Here's how the part is built. I have some questions about the finished solid (model axes, mm). A direction names the side the tool comes from. Coordinates: 2 decimals unless noted, no trailing zeros. Write each loop counter-clockwise with the first axis right and the second up, starting at its lowest first coordinate (ties: lowest second). Pieces come first, ordered by that corner, then holes. Notation, with made-up numbers: (0, -16.75) -> (26, -16.75) arc R16 ccw to (26, 1.25) -> close; hole circle Ø3 at (24, 88). An arc over 180 degrees is marked (long way). Use a Markdown table: item, result. Add a question column.
```python
from build123d import *

# Parameters (mm, degrees)
F0_R      = 12
F1_DEPTH  = 100
F2_R      = 10
F3_DEPTH  = 100
F4_R      = 32
F4_R_2    = 12
F5_DEPTH  = 5
F6_R      = 32
F6_R_2    = 12
F7_DEPTH  = 5
F8_R      = 5
F9_DEPTH  = 100
F14_R     = 5
F15_DEPTH = 50
F16_R     = 10
F17_DEPTH = 70


with BuildPart() as f1:
    # F0 (on Top) → F1 (new body)
    with BuildSketch(Plane.XY):
        Circle(F0_R)
    extrude(amount=F1_DEPTH)

    # F2 (on face) → F3 (cut, through all)
    with BuildSketch(Plane.XY.offset(100)):
        Circle(F2_R)
    extrude(amount=-F3_DEPTH, mode=Mode.SUBTRACT)

    # F4 (on face) → F5 (join)
    with BuildSketch(Plane(origin=(0, 0, 0), x_dir=(1, 0, 0), z_dir=(0, 0, -1))):
        Circle(F4_R)
        Circle(F4_R_2, mode=Mode.SUBTRACT)
    extrude(amount=-F5_DEPTH)

    # F6 (on face) → F7 (join)
    with BuildSketch(Plane.XY.offset(100)):
        Circle(F6_R)
        Circle(F6_R_2, mode=Mode.SUBTRACT)
    extrude(amount=-F7_DEPTH)

    # F8 (on face) → F9 (cut, through all)
    with BuildSketch(Plane.XY.offset(100)):
        with Locations((0, 20)):
            Circle(F8_R)
        with Locations((-20, 0)):
            Circle(F8_R)
        with Locations((0, -20)):
            Circle(F8_R)
        with Locations((20, 0)):
            Circle(F8_R)
    extrude(amount=-F9_DEPTH, mode=Mode.SUBTRACT)

    # F13: sweep along a path in F12
    with BuildLine(Plane.XZ.offset(5)) as f13_path:
        Line((0, 50), (50, 50))
    # F10 (on Right) → F13 (sweep)
    with BuildSketch(Plane.YZ):
        with BuildLine():
            ThreePointArc((0, 46.6833752096), (0.7445626465, 48.2679491924), (1, 50))
            ThreePointArc((1, 50), (-10.7445626465, 51.7320508076), (0, 46.6833752096))
        make_face()
    sweep(path=f13_path.line)

    # F14 (on face) → F15 (cut, through all)
    with BuildSketch(Plane.YZ.offset(50)):
        with Locations((-5, 50)):
            Circle(F14_R)
    extrude(amount=-F15_DEPTH, mode=Mode.SUBTRACT)

    # F16 (on face) → F17 (cut)
    with BuildSketch(Plane.XY.offset(100)):
        Circle(F16_R)
    extrude(amount=-F17_DEPTH, mode=Mode.SUBTRACT)


solid = f1.part
```
Q1. Suppose I cut it at A-A, the plane x = 20. Write out the boundary of the cut face in (y, z).
Q2. Thinking about a two-plate mould opening in X: for faces 1 (the cylindrical face through (-6.94, -31.24, 97.54)), 2 (the flat face through (14, 0, 5)), 3 (the cylindrical face through (15, 0, 3)), which applies, released by +X, released by -X, zero draft, split by the parting line, or undercut?
Q3. Will these pins go through, and if not, where does the flat tip stop? pin 1 (6 mm diameter, centred on x = 20, y = 0, fed in from +Z); pin 2 (6 mm diameter, centred on y = -5.5, z = 18.5, fed in from -X); pin 3 (9 mm diameter, centred on x = 20, y = 0, fed in from -Z).
Q4. Suppose I cut it at B-B, the plane x = -20. Write out the boundary of the cut face in (y, z), and give its area (3 significant figures).
Q5. Please list where these lines run through material, in increasing order: line 1 (Y direction, x = 0, z = 1); line 2 (Z direction, x = 15, y = -27); line 3 (Y direction, x = 30, z = 50).
Q6. Which directions (+Z, -Z, +X, -X, +Y, -Y) give clear straight access to the entire face, cutting with the end or side of a thin tool? Please do faces 4 (the cylindrical face through (15, 0, 98)), 5 (the cylindrical face through (-8.844, 8.11, 49.37)), 6 (the cylindrical face through (31, -10, 50)).
Q7. Suppose I cut it at D-D, the plane x = 3.5. State how many separate pieces and enclosed holes the cut face has, and give its area (3 significant figures).
Answer key:
| question | item | result |
|---|---|---|
| 1 | outline | (-24.98, 0) -> (-5, 0) -> (-5, 5) -> (-24.98, 5) -> close; (-24.98, 95) -> (-5, 95) -> (-5, 100) -> (-24.98, 100) -> close; circle Ø12 at (-5, 50); (5, 0) -> (24.98, 0) -> (24.98, 5) -> (5, 5) -> close; (5, 95) -> (24.98, 95) -> (24.98, 100) -> (5, 100) -> close; hole circle Ø10 at (-5, 50) |
| 2 | face 1 | split by the parting line |
| 2 | face 2 | zero draft |
| 2 | face 3 | undercut |
| 3 | pin 1 | stops at z = 55.66 |
| 3 | pin 2 | stops at x = -11.74 |
| 3 | pin 3 | stops at z = 44.02 |
| 4 | outline | (-24.98, 0) -> (-5, 0) -> (-5, 5) -> (-24.98, 5) -> close; (-24.98, 95) -> (-5, 95) -> (-5, 100) -> (-24.98, 100) -> close; (5, 0) -> (24.98, 0) -> (24.98, 5) -> (5, 5) -> close; (5, 95) -> (24.98, 95) -> (24.98, 100) -> (5, 100) -> close |
| 4 | area | 400 mm^2 |
| 5 | line 1 | y = -32 to -25, -15 to -10, 10 to 15, 25 to 32 |
| 5 | line 2 | z = 0 to 5, 95 to 100 |
| 5 | line 3 | y = -11 to -10, 0 to 1 |
| 6 | face 4 | +Z |
| 6 | face 5 | none |
| 6 | face 6 | +X |
| 7 | separate pieces | 6 |
| 7 | enclosed holes | 0 |
| 7 | area | 684 mm^2 |
